Build history of the part. All positions in model axes, mm. A direction names the side the tool comes from. Round coordinates to 2 decimals unless told otherwise and drop trailing zeros. Write each loop counter-clockwise with the first axis right and the second up, starting at its lowest first coordinate (ties: lowest second). Pieces come first, ordered by that corner, then holes. Notation, with made-up numbers: M 88.5,74 L 106.5,74 A23 cw 106.5,82 Z; hole C 65,78 d2. An arc over 180 degrees is marked long. Write item = value, one per line. Start each with the question number.
Q1. Band-saw the part on D-D on y = 1.5. Write the cut outline in (x, z).
Q2. Band-saw the part on A-A on y = 5.5. Write the cut outline in (x, z).
Q3. Band-saw the part on B-B on z = -3. Write the cut outline in (x, y), plus the area to 3 significant figures.
Q4. Tool access for faces 1 (the flat face through (-4, 2, 4)), 2 (the flat face through (0, 3, 16)): list every direction of +Z, -Z, +X, -X, +Y, -Y with a clear straight run to the whole face (end or side of a thin tool).
Q5. Drop flat-ended pins along their axis: P1, Ø1.4, axis at y = 4, z = -16, coming from the -X side; P2, Ø4, axis at y = 4, z = 3, coming from the -X side (3 decimals); P3, Ø0.5, axis at y = 3.5, z = 8.5, coming from the +X side; P4, Ø2, axis at x = 16, z = -15.5, coming from the +Y side. Give the stop position or say it passes through.
Q6. Band-saw the part on C-C on z = 8. Write the cut outline in (x, y), plus the area to 3 significant figures.
Q7. Pull direction Z, two halves, no side cores. Call faces 3 (the flat face through (-0.99, 3.84, -18.04)), 4 (the flat face through (13.13, 3.84, -9.89)): released by +Z, released by -Z, zero draft, split by the parting line, or undercut.
Q8. Probe L1, parallel to Y at x = -14, z = 10; L2, parallel to X at y = 6, z = -16.3; L3, parallel to Y at x = 0.5, z = -17. List the from-to ranges inside material, lowest first.
```python
from build123d import *

# Parameters (mm, degrees)
SKETCH1_R           = 20
BOSS_EXTRUDE1_DEPTH = 7
SKETCH2_R           = 8.5
CUT_EXTRUDE1_DEPTH  = 5
SKETCH3_R           = 4.5
CUT_EXTRUDE2_DEPTH  = 30.137604569
SKETCH4_R           = 1
CUT_EXTRUDE3_DEPTH  = 4
CUT_EXTRUDE4_DEPTH  = 1.7


with BuildPart() as part:
    # Sketch1 → Boss-Extrude1 (new body)
    with BuildSketch(Plane(origin=(0, 0, 0), x_dir=(1, 0, 0), z_dir=(0, 1, 0))):
        with Locations(Location((0, 0, 0), (0, 0, 270))):
            Circle(SKETCH1_R)
    extrude(amount=BOSS_EXTRUDE1_DEPTH)

    # Sketch2 → Cut-Extrude1 (cut)
    with BuildSketch(Plane(origin=(0, 7, 0), x_dir=(1, 0, 0), z_dir=(0, 1, 0))):
        with Locations(Location((0, 0, 0), (0, 0, 270))):
            Circle(SKETCH2_R)
    extrude(amount=-CUT_EXTRUDE1_DEPTH, mode=Mode.SUBTRACT)

    # Sketch3 → Cut-Extrude2 (cut, through all)
    with BuildSketch(Plane(origin=(0, 7, 0), x_dir=(1, 0, 0), z_dir=(0, 1, 0))):
        with Locations(Location((0, 0, 0), (0, 0, 270))):
            Circle(SKETCH3_R)
    extrude(amount=-CUT_EXTRUDE2_DEPTH, mode=Mode.SUBTRACT)

    # Sketch4 → Cut-Extrude3 (cut)
    with BuildSketch(Plane(origin=(0, 7, 0), x_dir=(1, 0, 0), z_dir=(0, 1, 0))):
        with Locations(Location((0, 16.3, 0), (0, 0, 270))):
            Circle(SKETCH4_R)
        with Locations(Location((14.116214082, 8.15, 0), (0, 0, 270))):
            Circle(SKETCH4_R)
        with Locations(Location((14.116214082, -8.15, 0), (0, 0, 270))):
            Circle(SKETCH4_R)
        with Locations(Location((0, -16.3, 0), (0, 0, 270))):
            Circle(SKETCH4_R)
        with Locations(Location((-14.116214082, -8.15, 0), (0, 0, 270))):
            Circle(SKETCH4_R)
        with Locations(Location((-14.116214082, 8.15, 0), (0, 0, 270))):
            Circle(SKETCH4_R)
    extrude(amount=-CUT_EXTRUDE3_DEPTH, mode=Mode.SUBTRACT)

    # Sketch5 → Cut-Extrude4 (cut)
    with BuildSketch(Plane(origin=(0, 3, 0), x_dir=(1, 0, 0), z_dir=(0, 1, 0))):
        Polygon((12.116214082, 6.995299462), (14.116214082, 5.840598923), (16.116214082, 6.995299462), (16.116214082, 9.304700538), (14.116214082, 10.459401077), (12.116214082, 9.304700538), align=None)
        Polygon((0, 13.990598923), (2, 15.145299462), (2, 17.454700538), (0, 18.609401077), (-2, 17.454700538), (-2, 15.145299462), align=None)
        Polygon((12.116214082, -6.995299462), (12.116214082, -9.304700538), (14.116214082, -10.459401077), (16.116214082, -9.304700538), (16.116214082, -6.995299462), (14.116214082, -5.840598923), align=None)
        Polygon((0, -13.990598923), (-2, -15.145299462), (-2, -17.454700538), (0, -18.609401077), (2, -17.454700538), (2, -15.145299462), align=None)
        Polygon((-12.116214082, -6.995299462), (-14.116214082, -5.840598923), (-16.116214082, -6.995299462), (-16.116214082, -9.304700538), (-14.116214082, -10.459401077), (-12.116214082, -9.304700538), align=None)
        Polygon((-12.116214082, 6.995299462), (-12.116214082, 9.304700538), (-14.116214082, 10.459401077), (-16.116214082, 9.304700538), (-16.116214082, 6.995299462), (-14.116214082, 5.840598923), align=None)
    extrude(amount=CUT_EXTRUDE4_DEPTH, mode=Mode.SUBTRACT)


solid = part.part
```
Conclusion:
q1.outline = C 0,0 d40; hole C 0,0 d9
q2.outline = C 0,0 d40; hole C -14.12,-8.15 d2; hole C -14.12,8.15 d2; hole C 0,0 d17; hole C 0,-16.3 d2; hole C 0,16.3 d2; hole C 14.12,-8.15 d2; hole C 14.12,8.15 d2
q3.outline = M -19.77,0 L -3.35,0 L -3.35,2 L -7.95,2 L -7.95,7 L -19.77,7 Z; M 3.35,0 L 19.77,0 L 19.77,7 L 7.95,7 L 7.95,2 L 3.35,2 Z
q3.area = 184 mm^2
q4.face_1 = +Y
q4.face_2 = none
q5.P1 = -12.88
q5.P2 = -19.975
q5.P3 = 18.22
q5.P4 = through
q6.outline = M -18.33,0 L 18.33,0 L 18.33,7 L 15.1,7 L 15.1,4.7 L 16.12,4.7 L 16.12,3 L 12.12,3 L 12.12,4.7 L 13.13,4.7 L 13.13,7 L 2.87,7 L 2.87,2 L -2.87,2 L -2.87,7 L -13.13,7 L -13.13,4.7 L -12.12,4.7 L -12.12,3 L -16.12,3 L -16.12,4.7 L -15.1,4.7 L -15.1,7 L -18.33,7 Z
q6.area = 205 mm^2
q7.face_3 = undercut
q7.face_4 = undercut
q8.L1 = 0 to 3, 4.7 to 7
q8.L2 = -11.59 to -1, 1 to 11.59
q8.L3 = 0 to 3
